Build history of the part. All positions in model axes, mm. Face numbers are marked on the shaded views. A direction names the side the tool comes from. Round coordinates to 2 decimals unless told otherwise and drop trailing zeros. Write each loop counter-clockwise with the first axis right and the second up, starting at its lowest first coordinate (ties: lowest second). Pieces come first, ordered by that corner, then holes. Notation, with made-up numbers: M 35.25,-33.5 L 54.25,-33.5 A6 ccw 54.25,-26.5 Z; hole C -33,-28 d7. An arc over 180 degrees is marked long. Write item = value, one per line.
from build123d import *

# Parameters (mm, degrees)
SKETCH1_R               = 26
BOSS_EXTRUDE1_DEPTH     = 35
BOSS_EXTRUDE2_DEPTH     = 15
SKETCH5_R               = 26
BOSS_EXTRUDE3_DEPTH     = 80
CUT_EXTRUDE2_DEPTH      = 41
CUT_EXTRUDE2_DEPTH_BACK = 41


with BuildPart() as part:
    # Sketch1 → Boss-Extrude1 (new body, symmetric)
    with BuildSketch(Plane(origin=(0, 0, 0), x_dir=(1, 0, 0), z_dir=(0, 1, 0))):
        Circle(SKETCH1_R)
    extrude(amount=BOSS_EXTRUDE1_DEPTH, both=True)

    # Sketch3 → Boss-Extrude2 (add)
    with BuildSketch(Plane(origin=(0, 35, 0), x_dir=(1, 0, 0), z_dir=(0, 1, 0))):
        with BuildLine():
            Line((0, 40), (80, 40))
            ThreePointArc((80, 40), (120, 0), (80, -40))
            Line((80, -40), (0, -40))
            ThreePointArc((0, -40), (-40, 0), (0, 40))
        make_face()
    boss_extrude2 = extrude(amount=BOSS_EXTRUDE2_DEPTH)

    # Mirror2: Boss-Extrude2 across plane
    add(boss_extrude2.mirror(Plane.ZX))

    # Sketch5 → Boss-Extrude3 (add)
    with BuildSketch(Plane(origin=(0, 50, 0), x_dir=(1, 0, 0), z_dir=(0, 1, 0))):
        with Locations((80, 0)):
            Circle(SKETCH5_R)
    boss_extrude3 = extrude(amount=BOSS_EXTRUDE3_DEPTH)

    # Mirror3: Boss-Extrude3 across plane
    add(boss_extrude3.mirror(Plane.ZX))

    # Sketch6 → Cut-Extrude2 (cut, two sides)
    with BuildSketch(Plane.XY) as cut_extrude2_sk:
        Polygon((0, -50), (-40, -50), (-40, -46), align=None)
        Polygon((80, -35), (120, -35), (120, -39), align=None)
        Polygon((120, 39), (80, 35), (120, 35), align=None)
        Polygon((-40, 46), (0, 50), (-40, 50), align=None)
    extrude(amount=CUT_EXTRUDE2_DEPTH, mode=Mode.SUBTRACT)
    extrude(cut_extrude2_sk.sketch, amount=-CUT_EXTRUDE2_DEPTH_BACK, mode=Mode.SUBTRACT)


solid = part.part
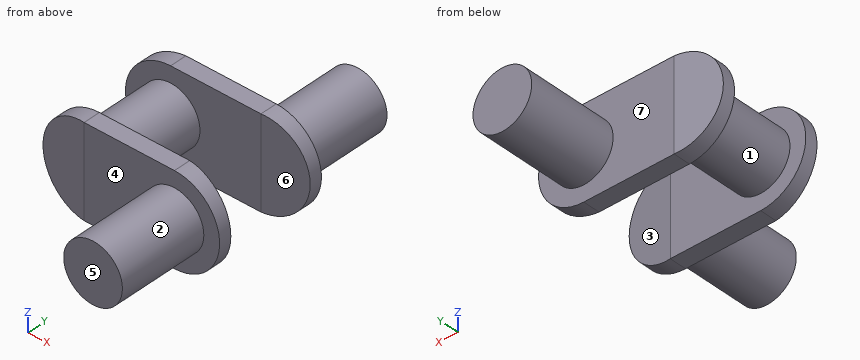
1. Probe probe 1 along Y at (x, z) = (34, -0.5); probe 2 along Y at (x, z) = (-17, 29.5); probe 3 along Z at (x, y) = (-1, 18.5). List the from-to ranges inside material, lowest first.
Responses:
probe_1 = -50 to -35, 35 to 50
probe_2 = -48.3 to -35, 35 to 48.3
probe_3 = -25.98 to 25.98
2. Band-saw the part on C-C (z = -31). List the corners of the cut face in (x, y).
Responses:
outline = M -25.28,-47.47 L 0,-50 L 105.28,-50 L 105.28,-37.53 L 80,-35 L -25.28,-35 Z; M -25.28,35 L 80,35 L 105.28,37.53 L 105.28,50 L 0,50 L -25.28,47.47 Z
3. Band-saw the part on D-D (y = 0). List the corners of the cut face in (x, z), plus the area to 3 significant figures.
Responses:
outline = C 0,0 d52
area = 2,120 mm²
4. Flat gauge pins, fed straight in: pin 1 (12 mm diameter, centred on x = 95.5, y = -103.5, fed in from +Z); pin 2 (1 mm diameter, centred on x = 17, z = 24.5, fed in from +Y); pin 3 (12 mm diameter, centred on x = -5.5, z = 11.5, fed in from -Y). Where does each tip first touch, or does it go through?
Responses:
pin_1 = 24.2
pin_2 = 50
pin_3 = -50
5. Mould opens along Y. For the marked faces 1, 2, 3 and 4 say: pulls with the +Y half, pulls with the -Y half, needs draft (parallel to the pull), parting line crosses it, or undercut.
Responses:
face_1 = undercut
face_2 = needs draft
face_3 = undercut
face_4 = pulls with the -Y half
6. Band-saw the part on A-A (x = 31). List the corners of the cut face in (y, z), plus the area to 3 significant figures.
Responses:
outline = M -50,-40 L -35,-40 L -35,40 L -50,40 Z; M 35,-40 L 50,-40 L 50,40 L 35,40 Z
area = 2,400 mm²
7. Band-saw the part on B-B (z = 0). List the corners of the cut face in (x, y).
Responses:
outline = M -40,-46 L 0,-50 L 54,-50 L 54,-130 L 106,-130 L 106,-50 L 120,-50 L 120,-39 L 80,-35 L 26,-35 L 26,35 L 80,35 L 120,39 L 120,50 L 106,50 L 106,130 L 54,130 L 54,50 L 0,50 L -40,46 L -40,35 L -26,35 L -26,-35 L -40,-35 Z
8. Tool access for the marked faces 5, 6 and 7: list every direction of +Z, -Z, +X, -X, +Y, -Y with a clear straight run to the whole face (end or side of a thin tool).
Responses:
face_5 = +Z, -Z, +X, -X, -Y
face_6 = +Z, -Z, +X
face_7 = +Y
